Read the model definition and answer for the solid it produces. Units are mm, in the model's axes. A direction names the side the tool comes from. Coordinates: 2 decimals unless noted, no trailing zeros. Write each loop counter-clockwise with the first axis right and the second up, starting at its lowest first coordinate (ties: lowest second). Pieces come first, ordered by that corner, then holes.
(1) Given pin 1 (5 mm diameter, centred on x = 22, z = 2.5, fed in from -Y); pin 2 (1 mm diameter, centred on x = 15, y = 2.5, fed in from -Z); pin 3 (8 mm diameter, centred on y = 0, z = 14, fed in from -X); pin 4 (5 mm diameter, centred on x = 21, z = 2, fed in from +Y), each flat-ended and moving along its own axis, determine where each tip first touches the part or whether it passes through.
(2) Which of the six approach directions +Z, -Z, +X, -X, +Y, -Y give full straight-line access (tool end or side, diameter ignored) to faces 4 (the cylindrical face through (28.619, -1.526, 4.845)), 5 (the cylindrical face through (2.123, 0.309, -0.251)), 6 (the cylindrical face through (8.675, 6.81, 16.424))?
(3) Straight lines are drawn through the part: line 1 along X through (y, z) = (-1, -4); line 2 along X through (y, z) = (1.5, 10) (3 decimals); line 3 along X through (y, z) = (12.5, 6.5) (3 decimals). For each, find the intervals that lie inside material, in ascending order.
(4) The part is cut by section A-A, the plane x = 13.5. Determine the outline of the cut face in (y, z), and give its area (3 significant figures).
(5) Determine the mould class of faces 1 (the cylindrical face through (11.134, 0.222, -0.251)), 2 (the flat face through (15.875, 8, 4)), 3 (the conical face through (25.32, 3.18, -4.14)) for opening direction Y: pulls with the +Y half, pulls with the -Y half, needs draft (parallel to the pull), parting line crosses it, or undercut.
(6) The part is cut by section B-B, the plane x = 17. Determine the outline of the cut face in (y, z) (1 decimal).
(7) The part is cut by section C-C, the plane y = 0. State how many separate pieces and enclosed holes the cut face has, and give its area (3 significant figures).
```python
from build123d import *

# Parameters (mm, degrees)
F_29_0_136_DIAMETER_HOLE1_D     = 3.4544
F_7_64_0_10938_DIAMETER_HOLE1_D = 2.778252
F_3_16_0_1875_DIAMETER_HOLE1_D  = 4.7625
FILLET1_R                       = 1.27


with BuildPart() as part:
    # Sketch1 → Revolve1 (revolve)
    with BuildSketch(Plane.XY, mode=Mode.PRIVATE) as revolve1_sk:
        Polygon((0, 0), (0, 17.78), (15.875, 17.78), (15.875, 7.9375), (23.750221606, 7.9375), (25.4, 5.08), (31.75, 5.08), (31.75, 0), (9.963821138, 0), align=None)
    revolve(revolve1_sk.sketch.rotate(Axis((-88.99, 0, 0), (1, 0, 0)), 90), axis=Axis((-88.99, 0, 0), (1, 0, 0)))

    # 29 _0.136_ Diameter Hole1 (through all)
    with Locations(Plane(origin=(12.84650937, 0.170730154, 17.779180274), x_dir=(0, 0.999953896174, -0.009602370845), z_dir=(0, 0.009602370845, 0.999953896174))):
        with Locations((0, 0)):
            Hole(F_29_0_136_DIAMETER_HOLE1_D / 2)

    # 7_64 _0.10938_ Diameter Hole1 (through all)
    with Locations(Plane(origin=(29.324260763, 0.062415003, 5.079616557), x_dir=(0, 0.99992451912, -0.012286417829), z_dir=(0, 0.012286417829, 0.99992451912))):
        with Locations((0, 0)):
            Hole(F_7_64_0_10938_DIAMETER_HOLE1_D / 2)

    # 3_16 _0.1875_ Diameter Hole1 (through all)
    with Locations(Plane(origin=(4.483845062, 0.076447724, 17.77983565), x_dir=(0, 0.999990756475, -0.004299647026), z_dir=(0, 0.004299647026, 0.999990756475))):
        with Locations((0, 0)):
            Hole(F_3_16_0_1875_DIAMETER_HOLE1_D / 2)

    # Fillet1
    fillet1_edges = [part.edges().sort_by_distance(p)[0] for p in [
        (0, 0, -17.78),
    ]]
    fillet(fillet1_edges, radius=FILLET1_R)


solid = part.part
```
Computed:
1. pin 1: stops at y = -7.94
1. pin 2: stops at z = -17.67
1. pin 3: stops at x = 0
1. pin 4: stops at y = 7.94
2. face 4: +X
2. face 5: none
2. face 6: +X, -X
3. line 1: x = 0 to 2.31, 6.65 to 11.41, 14.28 to 28.31, 30.34 to 31.75
3. line 2: x = 0 to 2.6, 6.367 to 11.84, 13.853 to 15.875
3. line 3: x = 0 to 15.875
4. outline: (-1.77, -17.69) - (-1.43, 17.72) arc R17.78 ccw to start; (1.43, -17.72) arc R17.78 ccw to (1.77, 17.69) - close
4. area: 880 mm2
5. face 1: undercut
5. face 2: needs draft
5. face 3: parting line crosses it
6. outline: circle Ø15.9 at (0, 0)
7. separate pieces: 4
7. enclosed holes: 0
7. area: 455 mm2
